The listing builds one solid part. Answer for the finished solid, in the listing's coordinates (mm). A direction names the side the tool comes from. Coordinates: 2 decimals unless noted, no trailing zeros. Write each loop counter-clockwise with the first axis right and the second up, starting at its lowest first coordinate (ties: lowest second). Pieces come first, ordered by that corner, then holes. Notation, with made-up numbers: M 77,8.5 L 110,8.5 A17 ccw 110,24.5 Z; hole C 3.5,81.25 d2. An arc over 180 degrees is marked long. Answer as CSV lines item,"result". Start each with the question number.
```python
from build123d import *

# Parameters (mm, degrees)
F1_DEPTH = 10


with BuildPart() as f1:
    # F0 (on Right) → F1 (new body)
    with BuildSketch(Plane.YZ):
        Polygon((0, 9.2), (0, 0), (80, 0), (80, 9.9), (70, 9.9), (70, 9.8), (60, 9.8), (60, 9.7), (50, 9.7), (50, 9.6), (40, 9.6), (40, 9.5), (30, 9.5), (30, 9.4), (20, 9.4), (20, 9.3), (10, 9.3), (10, 9.2), align=None)
    extrude(amount=F1_DEPTH)


solid = f1.part
```
1) Which of the six approach directions +Z, -Z, +X, -X, +Y, -Y give full straight-line access (tool end or side, diameter ignored) to faces 1 (the face through (5, 5, 9.2)), 2 (the face through (5, 0, 5))?
2) Find the intervals of material crossed by line 1 (Z direction, x = 0.5, y = 56); line 2 (Z direction, x = 1.75, y = 42), in increasing order. Write a range as from..to.
3) The part is cut by section A-A (x = 5.75). Determine the outline of the cut face in (y, z).
4) Each of these flat-tipped pins is pushed along its axis until it touches: P1, Ø3, axis at x = 4.5, y = 14.5, coming from the +Z side; P2, Ø5, axis at x = 3, y = 23.5, coming from the +Z side; P3, Ø3, axis at x = 2.5, y = 53, coming from the -Z side; P4, Ø3, axis at x = 7, y = 63.5, coming from the +Z side. Where does it stop, or does it pass through?
5) The part is cut by section C-C (y = 57.5). Determine the outline of the cut face in (x, z), then the cut area to 3 significant figures.
6) The part is cut by section B-B (y = 34). Determine the outline of the cut face in (x, z), then the cut area to 3 significant figures.
Completed:
1,face 1,"+Z, +X, -X, -Y"
1,face 2,"+Z, -Z, +X, -X, -Y"
2,line 1,"0..9.7"
2,line 2,"0..9.6"
3,outline,"M 0,0 L 80,0 L 80,9.9 L 70,9.9 L 70,9.8 L 60,9.8 L 60,9.7 L 50,9.7 L 50,9.6 L 40,9.6 L 40,9.5 L 30,9.5 L 30,9.4 L 20,9.4 L 20,9.3 L 10,9.3 L 10,9.2 L 0,9.2 Z"
4,P1,"z = 9.3"
4,P2,"z = 9.4"
4,P3,"z = 0"
4,P4,"z = 9.8"
5,outline,"M 0,0 L 10,0 L 10,9.7 L 0,9.7 Z"
5,area,"97.0 mm²"
6,outline,"M 0,0 L 10,0 L 10,9.5 L 0,9.5 Z"
6,area,"95.0 mm²"
